CAD build for the part. Positions are in the model's coordinates, mm. Face numbers are marked on the shaded views. A direction names the side the tool comes from. Coordinates: 2 decimals unless noted, no trailing zeros. Loops run counter-clockwise (first coordinate to the right, second up) from the corner with the lowest first, then second, coordinate; pieces in that order, holes last. Notation, with made-up numbers: (48, 70) -> (107, 70) arc R9 cw to (107, 84) -> close; hole circle Ø5 at (21, 44). An arc over 180 degrees is marked (long way). Write item = value, one per line. Start each with the question number.
(1) Drill centre lines: line 1 (Y direction, x = 3.5, z = -0.75); line 2 (Z direction, x = 0, y = 31); line 3 (X direction, y = 11.5, z = -2). Where is each one in solid material? Low to high. Write a range as from..to.
(2) Band-saw the part on A-A (y = 30.5). Write the cut outline in (x, z).
(3) Tool access for the marked faces 1 and 2: list every direction of +Z, -Z, +X, -X, +Y, -Y with a clear straight run to the whole face (end or side of a thin tool).
(4) Flat gauge pins, fed straight in: P1, Ø2, axis at y = 21, z = 1, coming from the +X side; P2, Ø1.5, axis at y = 4, z = 3.5, coming from the -X side; P3, Ø5, axis at x = 3.5, y = 31, coming from the -Z side; P4, Ø1.5, axis at x = -4, y = 30, coming from the -Z side. Where does each tip first touch, or does it go through?
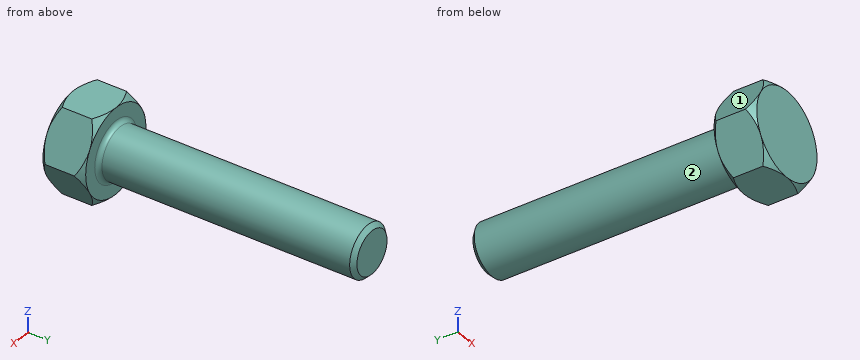
Autodesk Inventor part; units mm, degrees
ref_plane "YZ Plane" through (0, 0, 0) normal (1, 0, 0) x (0, 1, 0)
ref_plane "XZ Plane" through (0, 0, 0) normal (0, 1, 0) x (-1, 0, 0)
ref_plane "XY Plane" through (0, 0, 0) normal (0, 0, 1) x (1, 0, 0)
sketch "Esboço1" plane through (0, 0, 0) normal (0, 1, 0) x (-1, 0, 0)
  circle A0 centre (0, 0) radius 3
  line L0 (-2.8868, -5) -> (-5.7735, 0)
  line L1 (-5.7735, 0) -> (-2.8868, 5)
  line L2 (-2.8868, 5) -> (2.8868, 5)
  line L3 (2.8868, 5) -> (5.7735, 0)
  line L4 (5.7735, 0) -> (2.8868, -5)
  line L5 (2.8868, -5) -> (-2.8868, -5)
  dimension "d0" = 6
extrude "Extrusão1" add sketch "Esboço1" along normal blind 5
sketch "Esboço2" plane through (0, 0, 0) normal (1, 0, 0) x (0, 1, 0)
  point P0 (0, 0)
chamfer "Chanfro1" distance 0.5 angle 45 2 edges at (3, 0, 0) (3, 5, 0)
sketch "Esboço5" plane through (0, 0, 0) normal (0, -1, 0) x (1, 0, 0)
  circle A0 centre (0, 0) radius 5
extrude "Extrusão2" cut sketch "Esboço5" against normal through all draft 45 keep common part
sketch "Esboço6" plane through (0, 5, 0) normal (0, 1, 0) x (1, 0, 0)
  circle A0 centre (0, 0) radius 5
extrude "Extrusão3" cut sketch "Esboço6" against normal through all draft 45 keep common part
sketch "Esboço7" plane through (0, 5, 0) normal (0, 1, 0) x (1, 0, 0)
  circle A0 centre (0, 0) radius 3.5
extrude "Extrusão4" add sketch "Esboço7" against normal blind 5
sketch "Esboço8" plane through (0, 5, 0) normal (0, 1, 0) x (1, 0, 0)
  circle A0 centre (0, 0) radius 3
  dimension "d16" = 6
extrude "Extrusão5" add sketch "Esboço8" along normal blind 30
chamfer "Chanfro2" distance 0.5 angle 45 1 edges at (-3, 35, 0)
fillet "Arredondamento1" radius 0.5 1 edges at (-3, 5, 0)
thread "Rosca2"
properties part number "porca m6" material "Aço inoxidável"
Findings below:
q1.line_1 = 0..5
q1.line_2 = -3..3
q1.line_3 = -2.24..2.24
q2.outline = circle Ø6 at (0, 0)
q3.face_1 = +Z, -X, +Y, -Y
q3.face_2 = +Y
q4.P1 = 3
q4.P2 = -4.19
q4.P3 = -2.83
q4.P4 = through
